Read the model definition and answer for the solid it produces. Units are mm, in the model's axes. Face numbers are marked on the shaded views. A direction names the side the tool comes from. Round coordinates to 2 decimals unless told otherwise and drop trailing zeros. Loops run counter-clockwise (first coordinate to the right, second up) from the corner with the lowest first, then second, coordinate; pieces in that order, holes last. Notation, with made-up numbers: (48.5, 1.25) - (53.5, 1.25) arc R21 cw to (53.5, 27.25) - close; hole circle Ø9 at (78, -7.5). An arc over 180 degrees is marked (long way). Answer as CSV lines item,"result".
```python
from build123d import *

# Parameters (mm, degrees)
F0_R     = 11.635
F0_R_2   = 11.3175
F1_DEPTH = 7
F2_R     = 4
F3_SIZE  = 1
F4_R     = 11.3175
F4_R_2   = 11.25
F4_R_3   = 11.635
F5_DEPTH = 7


with BuildPart() as f1:
    # F0 (on Top) → F1 (new body)
    with BuildSketch(Plane.XY):
        with BuildLine():
            Line((17.023025, 33.009872), (0, 45))
            Line((0, 45), (-17.023025, 33.009872))
            Line((-17.023025, 33.009872), (-9.861474, 11.302714))
            ThreePointArc((-9.861474, 11.302714), (0, 15), (9.861474, 11.302714))
            Line((9.861474, 11.302714), (17.023025, 33.009872))
        make_face()
        with Locations((0, 27.524821)):
            Circle(F0_R, mode=Mode.SUBTRACT)
        with BuildLine():
            ThreePointArc((9.861474, 11.302714), (0, 15), (-9.861474, 11.302714))
            ThreePointArc((-9.861474, 11.302714), (-12.990381, 7.5), (-14.719174, 2.88893))
            ThreePointArc((-14.719174, 2.88893), (-12.990381, -7.5), (-4.8577, -14.191644))
            ThreePointArc((-4.8577, -14.191644), (0, -15), (4.8577, -14.191644))
            ThreePointArc((4.8577, -14.191644), (12.203801, -8.721654), (15, 0))
            ThreePointArc((15, 0), (14.929628, 1.451273), (14.719174, 2.88893))
            ThreePointArc((14.719174, 2.88893), (12.990381, 7.5), (9.861474, 11.302714))
        make_face()
        Circle(F0_R_2, mode=Mode.SUBTRACT)
        with BuildLine():
            ThreePointArc((-4.8577, -14.191644), (-12.990381, -7.5), (-14.719174, 2.88893))
            Line((-14.719174, 2.88893), (-37.0989, -1.762564))
            Line((-37.0989, -1.762564), (-38.971143, -22.5))
            Line((-38.971143, -22.5), (-20.075875, -31.247308))
            Line((-20.075875, -31.247308), (-4.8577, -14.191644))
        make_face()
        with Locations((-23.837195, -13.762411)):
            Circle(F0_R, mode=Mode.SUBTRACT)
        with BuildLine():
            Line((37.0989, -1.762564), (14.719174, 2.88893))
            ThreePointArc((14.719174, 2.88893), (14.929628, 1.451273), (15, 0))
            ThreePointArc((15, 0), (12.203801, -8.721654), (4.8577, -14.191644))
            Line((4.8577, -14.191644), (20.075875, -31.247308))
            Line((20.075875, -31.247308), (38.971143, -22.5))
            Line((38.971143, -22.5), (37.0989, -1.762564))
        make_face()
        with Locations((23.837195, -13.762411)):
            Circle(F0_R, mode=Mode.SUBTRACT)
    extrude(amount=F1_DEPTH)

    # F2
    f2_edges = [f1.edges().sort_by_distance(p)[0] for p in [
        (-20.075875, -31.247308, 3.5),
        (20.075875, -31.247308, 3.5),
        (38.971143, -22.5, 3.5),
        (37.0989, -1.762564, 3.5),
        (14.719174, 2.88893, 3.5),
        (9.861474, 11.302714, 3.5),
        (17.023025, 33.009872, 3.5),
        (0, 45, 3.5),
        (-17.023025, 33.009872, 3.5),
        (-9.861474, 11.302714, 3.5),
        (-14.719174, 2.88893, 3.5),
        (-37.0989, -1.762564, 3.5),
        (-38.971143, -22.5, 3.5),
        (-4.8577, -14.191644, 3.5),
        (4.8577, -14.191644, 3.5),
    ]]
    fillet(f2_edges, radius=F2_R)

    # F3
    f3_edges = [f1.edges().sort_by_distance(p)[0] for p in [
        (-13.359963, 21.906877, 7),
        (-13.359963, 21.906877, 0),
    ]]
    chamfer(f3_edges, length=F3_SIZE)

    # F4 (on face) → F5 (join)
    with BuildSketch(Plane.XY.offset(7)):
        Circle(F4_R)
        Circle(F4_R_2, mode=Mode.SUBTRACT)
        with Locations((0, 27.524821)):
            Circle(F4_R_3)
        with Locations((0, 27.524821)):
            Circle(F4_R_2, mode=Mode.SUBTRACT)
        with Locations((-23.837195, -13.762411)):
            Circle(F4_R_3)
        with Locations((-23.837195, -13.762411)):
            Circle(F4_R_2, mode=Mode.SUBTRACT)
        with Locations((23.837195, -13.762411)):
            Circle(F4_R_3)
        with Locations((23.837195, -13.762411)):
            Circle(F4_R_2, mode=Mode.SUBTRACT)
    extrude(amount=-F5_DEPTH)


solid = f1.part
```
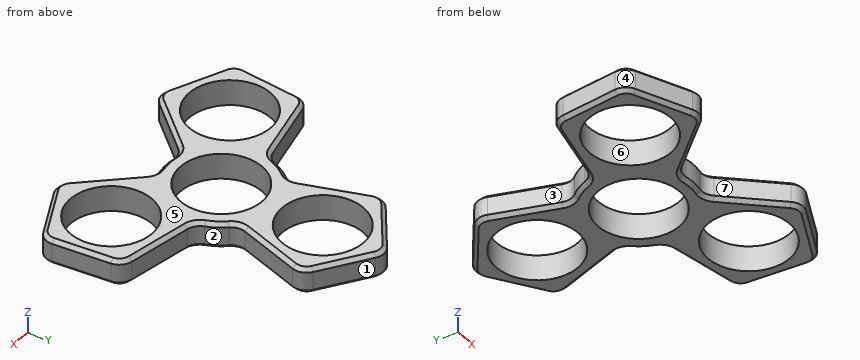
1) A cutting plane is placed at D-D, the plane z = 3.25. Count the separate pieces of the cut face and the enclosed holes in it, plus the area to 3 significant figures.
Entries:
separate pieces,"1"
enclosed holes,"4"
area,"1,320 mm^2"
2) The mould has two halves that part along X. Classify the marked faces 4, 5, 6 and 7: pulls with the +X half, pulls with the -X half, needs draft (parallel to the pull), parting line crosses it, or undercut.
Entries:
face 4,"pulls with the -X half"
face 5,"needs draft"
face 6,"undercut"
face 7,"undercut"
3) A cutting plane is placed at C-C, the plane y = 18. Determine the outline of the cut face in (x, z).
Entries:
outline,"(-12.07, 1) - (-11.02, 0) - (-5.99, 0) - (-5.99, 7) - (-11.02, 7) - (-12.07, 6) - close; (5.99, 0) - (11.02, 0) - (12.07, 1) - (12.07, 6) - (11.02, 7) - (5.99, 7) - close"
4) Find the intervals of material crossed by line 1 (Y direction, x = 0, z = 1.5); line 2 (X direction, y = -10, z = 2.25); line 3 (Y direction, x = -5.5, z = 1.75), in increasing order.
Entries:
line 1,"y = -15 to -11.25, 11.25 to 16.27, 38.77 to 44.11"
line 2,"x = -37.84 to -34.44, -13.23 to -5.15, 5.15 to 13.23, 34.44 to 37.84"
line 3,"y = -15.21 to -9.81, 9.81 to 17.71, 37.34 to 41.13"
5) Each of these flat-tipped pins is pushed along its axis until it touches: P1, Ø3, axis at y = 6.5, z = 6, coming from the +X side; P2, Ø20, axis at x = 0, y = 27.52, coming from the -Z side; P3, Ø1, axis at x = 15.5, z = 2, coming from the +Y side. Where does it stop, or does it pass through?
Entries:
P1,"stops at x = 14.14"
P2,"passes through"
P3,"stops at y = 34.39"
6) A tool of negligible diameter and unlimited length cuts with its end or side. For the marked faces 1, 2 and 3, from which of +Z, -Z, +X, -X, +Y, -Y can it reach the whole face along a straight path? Write none if from no direction.
Entries:
face 1,"+Z, -Z, +X, +Y"
face 2,"+Z, -Z, +X"
face 3,"+Z, -Z, -X"
7) A cutting plane is placed at A-A, the plane x = 0. Determine the outline of the cut face in (y, z), plus the area to 3 significant figures.
Entries:
outline,"(-15, 1) - (-14, 0) - (-11.25, 0) - (-11.25, 7) - (-14, 7) - (-15, 6) - close; (11.25, 0) - (16.27, 0) - (16.27, 7) - (11.25, 7) - close; (38.77, 0) - (43.11, 0) - (44.11, 1) - (44.11, 6) - (43.11, 7) - (38.77, 7) - close"
area,"96.8 mm^2"
8) A cutting plane is placed at B-B, the plane y = -6.5. Determine the outline of the cut face in (x, z), plus the area to 3 significant figures.
Entries:
outline,"(-37.53, 1) - (-36.52, 0) - (-32.43, 0) - (-32.43, 7) - (-36.52, 7) - (-37.53, 6) - close; (-15.25, 0) - (-9.18, 0) - (-9.18, 7) - (-15.25, 7) - close; (9.18, 0) - (15.25, 0) - (15.25, 7) - (9.18, 7) - close; (32.43, 0) - (36.52, 0) - (37.53, 1) - (37.53, 6) - (36.52, 7) - (32.43, 7) - close"
area,"154 mm^2"
